from build123d import *

# Parameters (mm, degrees)
F1_DEPTH = 25
F2_R     = 3
F3_R     = 1


with BuildPart() as f1:
    # F0 (on Front) → F1 (new body)
    with BuildSketch(Plane.XZ):
        Polygon((-25, 3.5), (-25, 0), (25, 0), (25, 3.5), (4.5, 3.5), (4.5, 23.5), (1, 23.5), (1, 3.5), (-1, 3.5), (-1, 23.5), (-4.5, 23.5), (-4.5, 3.5), align=None)
    extrude(amount=F1_DEPTH)

    # F2
    f2_edges = [f1.edges().sort_by_distance(p)[0] for p in [
        (-25, -25, 1.75),
        (-25, 0, 1.75),
        (-2.75, 0, 23.5),
        (-2.75, -25, 23.5),
        (2.75, -25, 23.5),
        (2.75, 0, 23.5),
        (25, -25, 1.75),
        (25, 0, 1.75),
    ]]
    fillet(f2_edges, radius=F2_R)

    # F3
    f3_edges = [f1.edges().sort_by_distance(p)[0] for p in [
        (-4.5, -12.5, 3.5),
        (4.5, -12.5, 3.5),
    ]]
    fillet(f3_edges, radius=F3_R)


solid = f1.part
Could you check a few things on this model? Use its own coordinates, in mm. A direction names the side the tool comes from. Give positions to 0.01 mm unless a question says otherwise; leave off trailing zeros. Order: outer loops, then holes, each group sorted by start corner. A loop starts at its lowest first (then second) coordinate and runs counter-clockwise, first axis right, second up. Notation, with made-up numbers: (-6, 0) -> (39, 0) arc R21 cw to (39, 26) -> close; hole circle Ø6 at (70, -1). An arc over 180 degrees is marked (long way). Answer in a Markdown table with one row per item. Add a question column.
Item 1: For faces 1 (the flat face through (4.5, -12, 14)), 2 (the flat face through (-15, -12, 3.5)), 3 (the cylindrical face through (-2.77, -0.9, 22.64)), 4 (the flat face through (-2, 0, 6)), 5 (the flat face through (0, -12, 3.5)), which set-ups out of +Z, -Z, +X, -X, +Y, -Y let a thin tool reach every point of the face, with its end or its side?
Item 2: Imagine slicing it at B-B (y = -16.5). List the corners of the cut face in (x, z) for me, and give its area (3 significant figures).
Item 3: Imagine slicing it at D-D (y = -2.5). List the corners of the cut face in (x, z) for me.
Item 4: Imagine slicing it at C-C (x = -10.5). List the corners of the cut face in (y, z) for me, and give its area (3 significant figures).
Item 5: Please list where these lines run through material, in increasing order: probe 1 along X at (y, z) = (-12.25, 22); probe 2 along Z at (x, y) = (-6, -19.5); probe 3 along Z at (x, y) = (-5, -11.5).
Item 6: Imagine slicing it at A-A (z = 9.5). List the corners of the cut face in (x, y) for me.
Item 7: I'm going to push flat-ended pins straight in: P1, Ø6, axis at y = -10, z = 11.5, coming from the +X side; P2, Ø6, axis at y = -18.5, z = 16.5, coming from the -X side; P3, Ø10, axis at x = 18, y = -16, coming from the +Z side. Where does each tip first touch, or does it pass through?
Result:
| question | item | result |
|---|---|---|
| 1 | face 1 | +Z, +X, +Y, -Y |
| 1 | face 2 | +Z, -X, +Y, -Y |
| 1 | face 3 | +Z, +X, -X, +Y |
| 1 | face 4 | +Z, -Z, +X, -X, +Y |
| 1 | face 5 | +Z, +Y, -Y |
| 2 | outline | (-25, 0) -> (25, 0) -> (25, 3.5) -> (5.5, 3.5) arc R1 cw to (4.5, 4.5) -> (4.5, 23.5) -> (1, 23.5) -> (1, 3.5) -> (-1, 3.5) -> (-1, 23.5) -> (-4.5, 23.5) -> (-4.5, 4.5) arc R1 cw to (-5.5, 3.5) -> (-25, 3.5) -> close |
| 2 | area | 315 mm2 |
| 3 | outline | (-24.96, 0) -> (24.96, 0) -> (24.96, 3.5) -> (5.5, 3.5) arc R1 cw to (4.5, 4.5) -> (4.5, 23.46) -> (1, 23.46) -> (1, 3.5) -> (-1, 3.5) -> (-1, 23.46) -> (-4.5, 23.46) -> (-4.5, 4.5) arc R1 cw to (-5.5, 3.5) -> (-24.96, 3.5) -> close |
| 4 | outline | (-25, 0) -> (0, 0) -> (0, 3.5) -> (-25, 3.5) -> close |
| 4 | area | 87.5 mm2 |
| 5 | probe 1 | -4.5 to -1, 1 to 4.5 |
| 5 | probe 2 | 0 to 3.5 |
| 5 | probe 3 | 0 to 3.63 |
| 6 | outline | (-4.5, -25) -> (-1, -25) -> (-1, 0) -> (-4.5, 0) -> close; (1, -25) -> (4.5, -25) -> (4.5, 0) -> (1, 0) -> close |
| 7 | P1 | x = 4.5 |
| 7 | P2 | x = -4.5 |
| 7 | P3 | z = 3.5 |
